Read the model definition and answer for the solid it produces. Units are mm, in the model's axes. A direction names the side the tool comes from. Round coordinates to 2 decimals unless told otherwise and drop trailing zeros. Order: outer loops, then holes, each group sorted by start corner. A loop starts at its lowest first (then second) coordinate and runs counter-clockwise, first axis right, second up. Notation, with made-up numbers: (-18, 83.5) -> (11, 83.5) arc R34 cw to (11, 114.5) -> close; hole circle Ø5 at (32.25, 80.25). An arc over 180 degrees is marked (long way). Answer as a JSON object with one key per item and string values. Group by question number.
Item 1: Consider probe 1 along X at (y, z) = (16, -7.5); probe 2 along Y at (x, z) = (-31, 6.75); probe 3 along Z at (x, y) = (-38.5, 1). Determine where each line is inside the solid, lowest interval first. Write a range as from..to.
Item 2: The mould has two halves that part along Y. Classify faces 4 (the cylindrical face through (43.3, -0.301, -9.287)), 5 (the cylindrical face through (45.13, -23.56, -1.9)), 6 (the flat face through (0, 23.868, 0)), 7 (the flat face through (46.552, -1, 0)): pulls with the +Y half, pulls with the -Y half, needs draft (parallel to the pull), parting line crosses it, or undercut.
Item 3: Section B-B, the plane z = -3.5 is taken. Write down the section's boundary in (x, y), plus the area to 3 significant figures.
Item 4: Given P1, Ø4, axis at x = -4.5, y = -2.5, coming from the +Z side; P2, Ø0.8, axis at y = 2.5, z = 11.5, coming from the -X side; P3, Ø2, axis at y = -6.5, z = 10.5, coming from the +X side, each flat-ended and moving along its own axis, determine where each tip first touches the part or whether it passes through.
Item 5: Section C-C, the plane y = 18 is taken. Write down the section's boundary in (x, z).
Item 6: Section A-A, the plane x = 12.5 is taken. Write down the section's boundary in (y, z).
Item 7: For faces 1 (the cylindrical face through (-43.4, -0.33, -11.07)), 2 (the flat face through (0, 18.868, 11)), 3 (the cylindrical face through (-41.648, -0.326, -9.287)), determine the directions among +Z, -Z, +X, -X, +Y, -Y from which every point of the face is accessible in a straight line to the end or side of a thin tool.
from build123d import *

# Parameters (mm, degrees)
F0_W         = 91.4515480399
F0_H         = 48.9329919219
F1_DEPTH     = 12.5
F2_R         = 5
F3_R         = 5
F4_T1_DEPTH  = 27.5
F4_T3_DEPTH  = 38.9329919219
F4_T5_DEPTH  = 81.4515480399
F4_S9_W      = 5.1
F4_S9_H      = 5.1
F4_T10_DEPTH = 5.1
F4_S15_W     = 5.1
F4_S15_H     = 5.1
F4_T16_DEPTH = 5.1
F4_T20_ANGLE = 90
F4_T22_ANGLE = 90
F5_T         = -2.5


# Not quite as in the source:
# - a fillet or chamfer that OpenCascade refuses, or shapes differently, is made with other operations: its cross-section is extruded or revolved along the edge and cut away or added
# - a shell that OpenCascade refuses in one call is made with other operations: the cavity is built on its own and cut out


with BuildPart() as f1:
    # F0 (on Top) → F1 (new body, symmetric)
    with BuildSketch(Plane.XY):
        with Locations((0.825881958, -0.5985237658)):
            Rectangle(F0_W, F0_H)
    extrude(amount=F1_DEPTH, both=True)

    # F2
    f2_edges = [f1.edges().sort_by_distance(p)[0] for p in [
        (-44.899892, 23.867972, 0),
    ]]
    fillet(f2_edges, radius=F2_R)

    # F3
    f3_edges = [f1.edges().sort_by_distance(p)[0] for p in [
        (-44.899892, -25.06502, 0),
        (3.325882, 23.867972, -12.5),
        (-43.435426, 22.403506, -12.5),
        (46.551656, -0.598524, -12.5),
        (-44.899892, -3.098524, -12.5),
        (0.825882, -25.06502, -12.5),
    ]]
    fillet(f3_edges, radius=F3_R)

    # F4: fillet of radius 5 on 9 edges, made by hand

    # F4_s2 → F4_t1 (cut)
    with BuildSketch(Plane.XY.offset(-20)):
        with BuildLine():
            ThreePointArc((41.551655978, 23.8679721951), (45.0871898839, 22.4035061011), (46.551655978, 18.8679721951))
            Line((46.551655978, 18.8679721951), (46.551655978, 23.8679721951))
            Line((46.551655978, 23.8679721951), (41.551655978, 23.8679721951))
        make_face()
        with BuildLine():
            ThreePointArc((46.551655978, -20.0650197268), (45.0871898839, -23.6005536327), (41.551655978, -25.0650197268))
            Line((41.551655978, -25.0650197268), (46.551655978, -25.0650197268))
            Line((46.551655978, -25.0650197268), (46.551655978, -20.0650197268))
        make_face()
    extrude(amount=F4_T1_DEPTH, mode=Mode.SUBTRACT)

    # F4_s4 → F4_t3 (cut)
    with BuildSketch(Plane.XZ.offset(-18.8679721951)):
        with BuildLine():
            ThreePointArc((41.551655978, 12.5), (45.0871898839, 11.0355339059), (46.551655978, 7.5))
            Line((46.551655978, 7.5), (46.551655978, 12.5))
            Line((46.551655978, 12.5), (41.551655978, 12.5))
        make_face()
        with BuildLine():
            ThreePointArc((-39.8998920619, 12.5), (-43.4354259679, 11.0355339059), (-44.8998920619, 7.5))
            Line((-44.8998920619, 7.5), (-44.8998920619, 12.5))
            Line((-44.8998920619, 12.5), (-39.8998920619, 12.5))
        make_face()
    extrude(amount=F4_T3_DEPTH, mode=Mode.SUBTRACT)

    # F4_s6 → F4_t5 (cut)
    with BuildSketch(Plane.YZ.offset(-39.8998920619)):
        with BuildLine():
            ThreePointArc((23.8679721951, 7.5), (22.4035061011, 11.0355339059), (18.8679721951, 12.5))
            Line((18.8679721951, 12.5), (23.8679721951, 12.5))
            Line((23.8679721951, 12.5), (23.8679721951, 7.5))
        make_face()
        with BuildLine():
            ThreePointArc((-20.0650197268, 12.5), (-23.6005536327, 11.0355339059), (-25.0650197268, 7.5))
            Line((-25.0650197268, 7.5), (-25.0650197268, 12.5))
            Line((-25.0650197268, 12.5), (-20.0650197268, 12.5))
        make_face()
    extrude(amount=F4_T5_DEPTH, mode=Mode.SUBTRACT)


with BuildPart() as f4_tool8:
    # F4_s9 → F4_t10 (new body)
    with BuildSketch(Plane.XZ.offset(-18.8679721951)):
        with Locations((44.101655978, 10.05)):
            Rectangle(F4_S9_W, F4_S9_H)
    extrude(amount=-F4_T10_DEPTH)

    # F4_s11 → F4_t12 (revolve, cut)
    with BuildSketch(Plane(origin=(41.551655978, 18.8679721951, 7.5), x_dir=(-0.7071067812, 0, -0.7071067812), z_dir=(0.7071067812, 0, -0.7071067812))):
        with BuildLine():
            ThreePointArc((0, -5), (5, 0), (0, 5))
            Line((0, 5), (0, -5))
        make_face()
    revolve(axis=Axis((41.551655978, 18.8679721951, 7.5), (0, 1, 0)), mode=Mode.SUBTRACT)


with BuildPart() as f1_1:
    add(f1.part)

    # F4_t7: cut F4_tool8
    add(f4_tool8.part, mode=Mode.SUBTRACT)


with BuildPart() as f4_tool14:
    # F4_s15 → F4_t16 (new body)
    with BuildSketch(Plane.XZ.offset(20.0650197268)):
        with Locations((44.101655978, 10.05)):
            Rectangle(F4_S15_W, F4_S15_H)
    extrude(amount=F4_T16_DEPTH)

    # F4_s17 → F4_t18 (revolve, cut)
    with BuildSketch(Plane(origin=(41.551655978, -20.0650197268, 7.5), x_dir=(-0.7071067812, 0, -0.7071067812), z_dir=(-0.7071067812, 0, 0.7071067812))):
        with BuildLine():
            ThreePointArc((0, -5), (5, 0), (0, 5))
            Line((0, 5), (0, -5))
        make_face()
    revolve(axis=Axis((41.551655978, -20.0650197268, 7.5), (0, -1, 0)), mode=Mode.SUBTRACT)


with BuildPart() as f1_2:
    add(f1_1.part)

    # F4_t13: cut F4_tool14
    add(f4_tool14.part, mode=Mode.SUBTRACT)

    # F4_s19 → F4_t20 (revolve, cut)
    with BuildSketch(Plane.YZ.offset(-39.8998920619)):
        with BuildLine():
            ThreePointArc((23.8679721951, 7.5), (22.4035061011, 11.0355339059), (18.8679721951, 12.5))
            Line((18.8679721951, 12.5), (23.8679721951, 12.5))
            Line((23.8679721951, 12.5), (23.8679721951, 7.5))
        make_face()
    revolve(axis=Axis((-39.8998920619, 18.8679721951, 12.5), (0, 0, 1)), revolution_arc=F4_T20_ANGLE, mode=Mode.SUBTRACT)

    # F4_s21 → F4_t22 (revolve, cut)
    with BuildSketch(Plane.XZ.offset(20.0650197268)):
        with BuildLine():
            ThreePointArc((-39.8998920619, 12.5), (-43.4354259679, 11.0355339059), (-44.8998920619, 7.5))
            Line((-44.8998920619, 7.5), (-44.8998920619, 12.5))
            Line((-44.8998920619, 12.5), (-39.8998920619, 12.5))
        make_face()
    revolve(axis=Axis((-39.8998920619, -20.0650197268, 12.5), (0, 0, 1)), revolution_arc=F4_T22_ANGLE, mode=Mode.SUBTRACT)

    # F5: a shell. OpenCascade refuses it in one call, so the cavity is built on its own and cut out:
    # the body offset inwards by the wall thickness, plus a prism from it out through each open face.
    f5_core = offset(f1_2.part, amount=F5_T, mode=Mode.PRIVATE)
    f5_exits = [f5_core.faces().sort_by_distance(p)[0] for p in [
        (0.825882, -0.598524, 10),
    ]]
    add(f5_core, mode=Mode.SUBTRACT)
    extrude(f5_exits, amount=-F5_T, mode=Mode.SUBTRACT)


solid = f1_2.part
Values found:
{
 "1": {"probe 1": "-44.9..-42.4, 44.05..46.55", "probe 2": "-25.07..-22.57, 21.37..23.87", "probe 3": "-12.5..-10"},
 "2": {"face 4": "undercut", "face 5": "pulls with the -Y half", "face 6": "pulls with the +Y half", "face 7": "needs draft"},
 "3": {"outline": "(-44.9, -20.07) arc R5 ccw to (-39.9, -25.07) -> (41.55, -25.07) arc R5 ccw to (46.55, -20.07) -> (46.55, 18.87) arc R5 ccw to (41.55, 23.87) -> (-39.9, 23.87) arc R5 ccw to (-44.9, 18.87) -> close; hole (-42.4, -20.07) arc R2.5 ccw to (-39.9, -22.57) -> (41.55, -22.57) arc R2.5 ccw to (44.05, -20.07) -> (44.05, 18.87) arc R2.5 ccw to (41.55, 21.37) -> (-39.9, 21.37) arc R2.5 ccw to (-42.4, 18.87) -> close", "area": "661 mm2"},
 "4": {"P1": "z = -10", "P2": "x = -43.37", "P3": "x = 46.13"},
 "5": {"outline": "(-44.9, -7.5) arc R5 ccw to (-39.9, -12.5) -> (41.55, -12.5) arc R5 ccw to (46.55, -7.5) -> (46.55, 7.5) arc R5 ccw to (41.55, 12.5) -> (41.55, 10) arc R2.5 cw to (44.05, 7.5) -> (44.05, -7.5) arc R2.5 cw to (41.55, -10) -> (-39.9, -10) arc R2.5 cw to (-42.4, -7.5) -> (-42.4, 7.5) arc R2.5 cw to (-39.9, 10) -> (-39.9, 12.5) arc R5 ccw to (-44.9, 7.5) -> close"},
 "6": {"outline": "(-25.07, -7.5) arc R5 ccw to (-20.07, -12.5) -> (18.87, -12.5) arc R5 ccw to (23.87, -7.5) -> (23.87, 7.5) arc R5 ccw to (18.87, 12.5) -> (18.87, 10) arc R2.5 cw to (21.37, 7.5) -> (21.37, -7.5) arc R2.5 cw to (18.87, -10) -> (-20.07, -10) arc R2.5 cw to (-22.57, -7.5) -> (-22.57, 7.5) arc R2.5 cw to (-20.07, 10) -> (-20.07, 12.5) arc R5 ccw to (-25.07, 7.5) -> close"},
 "7": {"face 1": "-Z, -X, +Y, -Y", "face 2": "+Z", "face 3": "none"}
}
